Here's how the part is built. I have some questions about the finished solid (model axes, mm). Face numbers are marked on the shaded views. A direction names the side the tool comes from. Round coordinates to 2 decimals unless told otherwise and drop trailing zeros. Write each loop counter-clockwise with the first axis right and the second up, starting at its lowest first coordinate (ties: lowest second). Pieces come first, ordered by that corner, then holes. Notation, with made-up numbers: M -31.5,5 L -21.5,5 A20 cw -21.5,32 Z; hole C 54.25,-32 d11. An arc over 180 degrees is marked long. Use one line per item in the form item = value. Start each with the question number.
Q1. For the marked faces 4, 5 and 6, which set-ups out of +Z, -Z, +X, -X, +Y, -Y let a thin tool reach every point of the face, with its end or its side?
Q2. We'd pull the mould along Z, two halves only. Please class the marked faces 1, 2 and 3: +Z half, -Z half, draft (parallel to the pull), parting line (faces both ways), or undercut.
Q3. I want a section at B-B on x = 20. List the corners of the cut face in (y, z) for me, and give its area (3 significant figures).
Q4. I'm going to push flat-ended pins straight in: pin 1 Ø0.7 at (y, z) = (-2.5, -26) entering from +X; pin 2 Ø3 at (x, y) = (19, -2.5) entering from -Z; pin 3 Ø1 at (x, y) = (32.5, -3) entering from +Z. Where does each tip first touch, or does it pass through?
Q5. I need wall thicknesses on line 1 along Z through (x, y) = (22.5, -7.25); line 2 along X through (y, z) = (3.75, -5.5); line 3 along Y through (x, z) = (30, -10). Which ranges of each line are inside material? Lowest first, please. Write a range as from..to.
Q6. I want a section at D-D on y = -7.25. List the corners of the cut face in (x, z) for me, and give its area (3 significant figures).
Q7. I want a section at C-C on z = -9. List the corners of the cut face in (x, y) for me.
Q8. I want a section at A-A on y = 3.25. List the corners of the cut face in (x, z) for me, and give its area (3 significant figures).
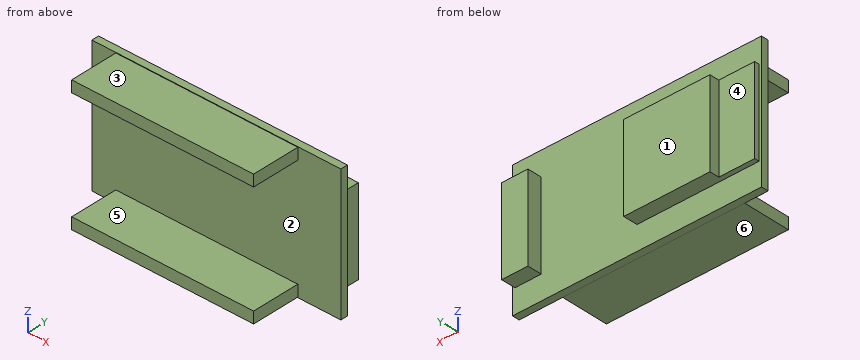
Autodesk Inventor part; units mm, degrees
ref_plane "YZ Plane" through (0, 0, 0) normal (1, 0, 0) x (0, 1, 0)
ref_plane "XZ Plane" through (0, 0, 0) normal (0, 1, 0) x (-1, 0, 0)
ref_plane "XY Plane" through (0, 0, 0) normal (0, 0, 1) x (1, 0, 0)
sketch "Sketch1" plane through (0, 0, 0) normal (0, 1, 0) x (-1, 0, 0)
  line L0 (0, 0) -> (-52, 0)
  line L1 (-52, 0) -> (-52, -28)
  line L2 (-52, -28) -> (0, -28)
  line L3 (0, -28) -> (0, 0)
  dimension "d0" = 52
  dimension "d1" = 28
extrude "Extrusion1" add sketch "Sketch1" along normal blind 1.5
sketch "Sketch2" plane through (0, 1.5, 0) normal (0, 1, 0) x (1, 0, 0)
  line L0 (0, 0) -> (0, 5) construction
  line L1 (0, 28) -> (0, 0) construction
  line L2 (0, 28) -> (0, 23) construction
  line L3 (0, 23) -> (8, 23)
  line L4 (8, 23) -> (8, 5)
  line L5 (8, 5) -> (0, 5)
  line L6 (0, 5) -> (0, 23)
  dimension "d4" = 5
  dimension "d5" = 5
  dimension "d6" = 8
extrude "Extrusion2" add sketch "Sketch2" along normal blind 1
sketch "Sketch3" plane through (0, 1.5, 0) normal (0, 1, 0) x (1, 0, 0)
  line L0 (8, 5) -> (8, 23)
  line L1 (8, 23) -> (26, 23)
  line L2 (26, 23) -> (26, 5)
  line L3 (26, 5) -> (8, 5)
  line L4 (8, 5) -> (8, 23)
  point P0 (0, 0)
  dimension "d9" = 18
extrude "Extrusion3" add sketch "Sketch3" along normal blind 3
sketch "Sketch4" plane through (0, 1.5, 0) normal (0, 1, 0) x (1, 0, 0)
  line L0 (52, 28) -> (52, 23) construction
  line L1 (52, 0) -> (52, 28) construction
  line L2 (52, 0) -> (52, 5) construction
  line L3 (52, 23) -> (46, 23)
  line L4 (46, 23) -> (46, 5)
  line L5 (46, 5) -> (52, 5)
  line L6 (52, 5) -> (52, 23)
  point P0 (0, 0)
  dimension "d12" = 5
  dimension "d13" = 5
  dimension "d14" = 6
extrude "Extrusion4" add sketch "Sketch4" along normal blind 3
sketch "Sketch5" plane through (52, 0, 0) normal (1, 0, 0) x (0, 0, -1)
  line L0 (5, 4.5) -> (23, 4.5)
  line L1 (23, 1.5) -> (28, 1.5)
  line L2 (5, 4.5) -> (23, 4.5)
  line L3 (23, 4.5) -> (23, 1.5)
  line L4 (23, 1.5) -> (5, 1.5)
  line L5 (5, 1.5) -> (5, 4.5)
  point P0 (0, 0)
extrude "Extrusion5" cut sketch "Sketch5" against normal blind 0.5
sketch "Sketch6" plane through (0, 0, -28) normal (-1, 0, 0) x (0, 0, 1)
  line L0 (5, 2.5) -> (23, 2.5)
  line L1 (23, 1.5) -> (5, 1.5)
  line L2 (5, 2.5) -> (23, 2.5)
  line L3 (23, 2.5) -> (23, 1.5)
  line L4 (23, 1.5) -> (5, 1.5)
  line L5 (5, 1.5) -> (5, 2.5)
  point P0 (28, 0)
extrude "Extrusion6" cut sketch "Sketch6" against normal blind 0.5
sketch "Sketch7" plane through (0, 0, 0) normal (0, -1, 0) x (1, 0, 0)
  line L0 (0, -28) -> (0, 0) construction
  line L1 (0, 0) -> (5, 0) construction
  line L2 (0, 0) -> (52, 0) construction
  line L3 (52, 0) -> (43, 0) construction
  line L4 (5, 0) -> (43, 0)
  line L5 (43, 0) -> (43, -2.5)
  line L6 (43, -2.5) -> (5, -2.5)
  line L7 (5, -2.5) -> (5, 0)
  line L8 (52, -28) -> (0, -28)
  line L9 (5, -28) -> (43, -28)
  line L10 (43, -28) -> (43, -25.5)
  line L11 (43, -25.5) -> (5, -25.5)
  line L12 (5, -25.5) -> (5, -28)
  dimension "d21" = 5
  dimension "d22" = 9
  dimension "d23" = 2.5
  dimension "d24" = 2.5
extrude "Extrusion7" add sketch "Sketch7" along normal blind 10
sketch "Sketch8" plane through (52, 1.5, -28) normal (0, 0, -1) x (-1, 0, 0)
  line L0 (47, -11.5) -> (9, -11.5)
  line L1 (9, -1.5) -> (9, -11.5)
  line L2 (47, -11.5) -> (9, -11.5)
  line L3 (9, -11.5) -> (9, -1.5)
  line L4 (9, -1.5) -> (47, -1.5)
  line L5 (47, -1.5) -> (47, -11.5)
  point P0 (52, -1.5)
extrude "Extrusion8" cut sketch "Sketch8" against normal blind 0.1
sketch "Sketch9" plane through (0, 1.5, 0) normal (0, 0, 1) x (1, 0, 0)
  line L0 (5, -1.5) -> (5, -11.5)
  line L1 (43, -11.5) -> (43, -1.5)
  line L2 (5, -1.5) -> (43, -1.5)
  line L3 (43, -1.5) -> (43, -11.5)
  line L4 (43, -11.5) -> (5, -11.5)
  line L5 (5, -11.5) -> (5, -1.5)
  point P0 (0, -1.5)
extrude "Extrusion9" cut sketch "Sketch9" against normal blind 0.1
properties part number "ESP32"
Reported:
q1.face_4 = +Z, -Z, -X, +Y
q1.face_5 = +X, -X, -Y
q1.face_6 = -Z, +X, -X, -Y
q2.face_1 = draft
q2.face_2 = undercut
q2.face_3 = +Z half
q3.outline = M -10,-27.9 L 0,-27.9 L 0,-28 L 1.5,-28 L 1.5,-23 L 4.5,-23 L 4.5,-5 L 1.5,-5 L 1.5,0 L 0,0 L 0,-0.1 L -10,-0.1 L -10,-2.5 L 0,-2.5 L 0,-25.5 L -10,-25.5 Z
q3.area = 144 mm^2
q4.pin_1 = 43
q4.pin_2 = -27.9
q4.pin_3 = -0.1
q5.line_1 = -27.9..-25.5, -2.5..-0.1
q5.line_2 = 8..26, 46..51.5
q5.line_3 = 0..1.5
q6.outline = M 5,-27.9 L 43,-27.9 L 43,-25.5 L 5,-25.5 Z; M 5,-2.5 L 43,-2.5 L 43,-0.1 L 5,-0.1 Z
q6.area = 182 mm^2
q7.outline = M 0,0 L 52,0 L 52,1.5 L 51.5,1.5 L 51.5,4.5 L 46,4.5 L 46,1.5 L 26,1.5 L 26,4.5 L 8,4.5 L 8,2.5 L 0.5,2.5 L 0.5,1.5 L 0,1.5 Z
q8.outline = M 8,-23 L 26,-23 L 26,-5 L 8,-5 Z; M 46,-23 L 51.5,-23 L 51.5,-5 L 46,-5 Z
q8.area = 423 mm^2
